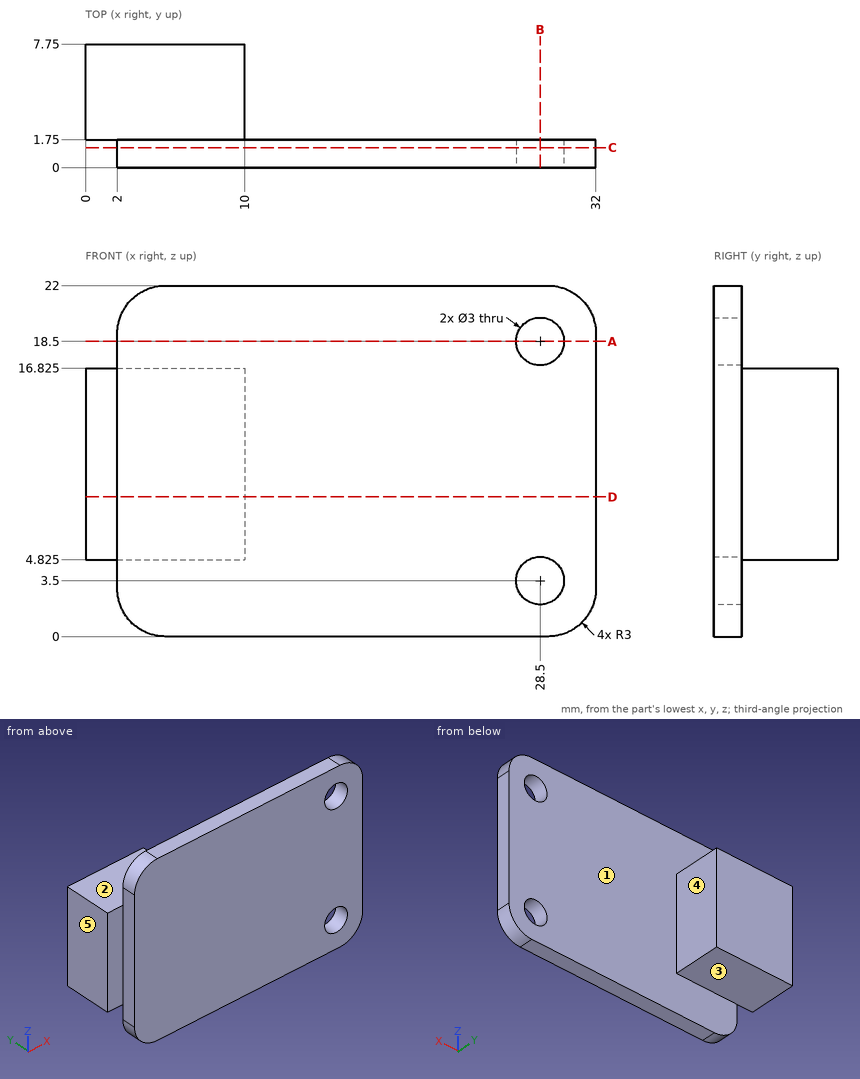
The drawing under review shows one solid part. Ordinate dimensions are in mm from its lowest x, y, z. A direction names the side the tool comes from. Coordinates: 2 decimals unless noted, no trailing zeros. Order: outer loops, then holes, each group sorted by start corner. A loop starts at its lowest first (then second) coordinate and runs counter-clockwise, first axis right, second up. Notation, with made-up numbers: (50, 3.25) -> (60, 3.25) arc R14 ccw to (60, 7.25) -> close; hole circle Ø10 at (-23, -15). An arc over 180 degrees is marked (long way). Answer in a Markdown table with one row per item. Add a question column.
Item 1: We need section B-B on x = 28.5. Write out the cut boundary in (y, z), plus the area to 3 significant figures.
Item 2: To check wall thickness, follow probe 1 along X at (y, z) = (0.45, 18.5); probe 2 along Z at (x, y) = (27.5, 1.5); probe 3 along Y at (x, z) = (7.5, 19). State the ranges of each line that lie inside material, in increasing order.
Item 3: We need section D-D on z = 8.75. Write out the cut boundary in (x, y).
Item 4: We need section A-A on z = 18.5. Write out the cut boundary in (x, y).
Item 5: Mouldability with a two-part tool opening along Z and no side actions: class the marked faces 1, 2 and 3 as +Z half, -Z half, draft (parallel to the pull), parting line (faces both ways), or undercut.
Item 6: Clearance check with flat-ended pins moving along their axes: pin 1 (3 mm diameter, centred on x = 3, y = 3.5, fed in from +Z) (3 decimals); pin 2 (6.5 mm diameter, centred on x = 13.5, z = 11, fed in from +Y); pin 3 (0.5 mm diameter, centred on y = 0.5, z = 7.5, fed in from -X). State where each tip first meets the part, or that it passes through.
Item 7: Machinability: for the marked faces 4 and 5, which of the approach directions +Z, -Z, +X, -X, +Y, -Y give a long, thin tool a straight path to every point of the face, cutting with its end or side? Answer none if there is none.
Item 8: We need section C-C on y = 1.25. Write out the cut boundary in (x, z).
Final values:
| question | item | result |
|---|---|---|
| 1 | outline | (0, 0) -> (1.75, 0) -> (1.75, 2) -> (0, 2) -> close; (0, 5) -> (1.75, 5) -> (1.75, 17) -> (0, 17) -> close; (0, 20) -> (1.75, 20) -> (1.75, 22) -> (0, 22) -> close |
| 1 | area | 28.0 mm2 |
| 2 | probe 1 | x = 2 to 27, 30 to 32 |
| 2 | probe 2 | z = 0 to 2.38, 4.62 to 17.38, 19.62 to 22 |
| 2 | probe 3 | y = 0 to 1.75 |
| 3 | outline | (0, 1.75) -> (2, 1.75) -> (2, 0) -> (32, 0) -> (32, 1.75) -> (10, 1.75) -> (10, 7.75) -> (0, 7.75) -> close |
| 4 | outline | (2, 0) -> (27, 0) -> (27, 1.75) -> (2, 1.75) -> close; (30, 0) -> (32, 0) -> (32, 1.75) -> (30, 1.75) -> close |
| 5 | face 1 | draft |
| 5 | face 2 | +Z half |
| 5 | face 3 | -Z half |
| 6 | pin 1 | stops at z = 16.825 |
| 6 | pin 2 | stops at y = 1.75 |
| 6 | pin 3 | stops at x = 2 |
| 7 | face 4 | +Z, -Z, +X, +Y |
| 7 | face 5 | +Z, -Z, -X, +Y, -Y |
| 8 | outline | (2, 3) arc R3 ccw to (5, 0) -> (29, 0) arc R3 ccw to (32, 3) -> (32, 19) arc R3 ccw to (29, 22) -> (5, 22) arc R3 ccw to (2, 19) -> close; hole circle Ø3 at (28.5, 3.5); hole circle Ø3 at (28.5, 18.5) |
